```python
from build123d import *

# Parameters (mm, degrees)
BOSS_EXTRUDE1_DEPTH  = 12.5
CUT_EXTRUDE1_START   = -10
SKETCH2_W            = 31
SKETCH2_H            = 10
CUT_EXTRUDE1_DEPTH   = 161.165360752
CUT_EXTRUDE2_DEPTH   = 10
CUT_EXTRUDE3_DEPTH   = 2
FILLET3_R            = 2
FILLET3_OF_MIRROR2_R = 2
SKETCH6_R            = 3
CUT_EXTRUDE5_DEPTH   = 164.267418673
FILLET4_R            = 3
FILLET4_OF_MIRROR3_R = 3


with BuildPart() as part:
    # Sketch1 → Boss-Extrude1 (new, symmetric)
    with BuildSketch(Plane(origin=(0, 0, 0), x_dir=(1, 0, 0), z_dir=(0, 1, 0))):
        Polygon((0, 120), (10, 120), (120, 10), (120, 0), (85, 0), (85, 9.644660941), (9.644660941, 85), (0, 85), align=None)
    extrude(amount=BOSS_EXTRUDE1_DEPTH, both=True)

    # Sketch2 → Cut-Extrude1 (cut, through all)
    with BuildSketch(Plane.XY.offset(CUT_EXTRUDE1_START)):
        with Locations((104.5, 0)):
            Rectangle(SKETCH2_W, SKETCH2_H)
    cut_extrude1 = extrude(amount=-CUT_EXTRUDE1_DEPTH, mode=Mode.SUBTRACT)

    # Sketch3 → Cut-Extrude2 (cut)
    with BuildSketch(Plane.XZ.offset(12.5)):
        Polygon((57.505379907, -44.210348845), (85, -16.715728753), (85, -37.928932188), align=None)
        Polygon((16.715728753, -85), (37.928932188, -85), (44.210348845, -57.505379907), align=None)
        Polygon((44.576447719, -78.352484469), (78.352484469, -44.576447719), (50.857864376, -50.857864376), align=None)
    cut_extrude2 = extrude(amount=-CUT_EXTRUDE2_DEPTH, mode=Mode.SUBTRACT)

    # Sketch4 → Cut-Extrude3 (cut)
    with BuildSketch(Plane.XZ.offset(12.5)):
        Polygon((5, -90), (32.928932188, -90), (7.928932188, -115), (5, -115), align=None)
        Polygon((115, -5), (90, -5), (90, -32.928932188), (115, -7.928932188), align=None)
    cut_extrude3 = extrude(amount=-CUT_EXTRUDE3_DEPTH, mode=Mode.SUBTRACT)

    # Fillet3
    fillet3_edges = [part.edges().sort_by_distance(p)[0] for p in [
        (16.715728753, -7.5, -85),
        (44.210348845, -7.5, -57.505379907),
        (37.928932188, -7.5, -85),
        (50.857864376, -7.5, -50.857864376),
        (78.352484469, -7.5, -44.576447719),
        (44.576447719, -7.5, -78.352484469),
        (85, -7.5, -37.928932188),
        (57.505379907, -7.5, -44.210348845),
        (85, -7.5, -16.715728753),
        (5, -11.5, -115),
        (5, -11.5, -90),
        (32.928932188, -11.5, -90),
        (7.928932188, -11.5, -115),
        (90, -11.5, -32.928932188),
        (90, -11.5, -5),
        (115, -11.5, -5),
        (115, -11.5, -7.928932188),
    ]]
    fillet(fillet3_edges, radius=FILLET3_R)

    # Mirror2: Cut-Extrude2, Cut-Extrude3 across plane
    add(cut_extrude2.mirror(Plane.ZX), mode=Mode.SUBTRACT)
    add(cut_extrude3.mirror(Plane.ZX), mode=Mode.SUBTRACT)

    # Fillet3 of Mirror2
    fillet3_of_mirror2_edges = [part.edges().sort_by_distance(p)[0] for p in [
        (16.715728753, 7.5, -85),
        (44.210348845, 7.5, -57.505379907),
        (37.928932188, 7.5, -85),
        (50.857864376, 7.5, -50.857864376),
        (78.352484469, 7.5, -44.576447719),
        (44.576447719, 7.5, -78.352484469),
        (85, 7.5, -37.928932188),
        (57.505379907, 7.5, -44.210348845),
        (85, 7.5, -16.715728753),
        (5, 11.5, -115),
        (5, 11.5, -90),
        (32.928932188, 11.5, -90),
        (7.928932188, 11.5, -115),
        (90, 11.5, -32.928932188),
        (90, 11.5, -5),
        (115, 11.5, -5),
        (115, 11.5, -7.928932188),
    ]]
    fillet(fillet3_of_mirror2_edges, radius=FILLET3_OF_MIRROR2_R)

    # Sketch6 → Cut-Extrude5 (cut, through all)
    with BuildSketch(Plane(origin=(0, 0, -10), x_dir=(-1, 0, 0), z_dir=(0, 0, -1))):
        with Locations((-113.5, 0)):
            Circle(SKETCH6_R)
        with Locations((-95.5, 0)):
            Circle(SKETCH6_R)
    cut_extrude5 = extrude(amount=-CUT_EXTRUDE5_DEPTH, mode=Mode.SUBTRACT)

    # Fillet4
    fillet4_edges = [part.edges().sort_by_distance(p)[0] for p in [
        (89, -5, -25.5),
        (89, 5, -25.5),
    ]]
    fillet(fillet4_edges, radius=FILLET4_R)

    # Mirror3: Cut-Extrude1, Cut-Extrude5 across plane
    add(cut_extrude1.mirror(Plane(origin=(0, 0, 0), x_dir=(-0.7071067811865475, 0, 0.7071067811865477), z_dir=(0.7071067811865476, 0, 0.7071067811865475))), mode=Mode.SUBTRACT)
    add(cut_extrude5.mirror(Plane(origin=(0, 0, 0), x_dir=(-0.7071067811865475, 0, 0.7071067811865477), z_dir=(0.7071067811865476, 0, 0.7071067811865475))), mode=Mode.SUBTRACT)

    # Fillet4 of Mirror3
    fillet4_of_mirror3_edges = [part.edges().sort_by_distance(p)[0] for p in [
        (25.5, -5, -89),
        (25.5, 5, -89),
    ]]
    fillet(fillet4_of_mirror3_edges, radius=FILLET4_OF_MIRROR3_R)


solid = part.part
```
CAD build for the part. Positions are in the model's coordinates, mm. A direction names the side the tool comes from. Round coordinates to 2 decimals unless told otherwise and drop trailing zeros. Order: outer loops, then holes, each group sorted by start corner. A loop starts at its lowest first (then second) coordinate and runs counter-clockwise, first axis right, second up.
Item 1: Saw through at A-A on y = 6.75. Write the cut outline in (x, z), then the cut area to 3 significant figures.
Item 2: Saw through at C-C on x = 95.5. Write the cut outline in (y, z).
Item 3: Saw through at B-B on z = -95.5. Write the cut outline in (x, y).
Item 4: Tool access for faces 5 (the face through (120, 0, -5)), 6 (the face through (5, 0, -85)), 7 (the face through (73.795, 7.43, -47.137)), 8 (the face through (103.77, -11.51, -19.16)), 9 (the face through (5.07, 0.9, -110.64)): list every direction of +Z, -Z, +X, -X, +Y, -Y with a clear straight run to the whole face (end or side of a thin tool).
Item 5: Pin check, flat tips, straight feed: pin 1 (8.5 mm diameter, centred on x = 17, z = -103, fed in from +Y); pin 2 (4 mm diameter, centred on x = 88, y = 3, fed in from -Z); pin 3 (1 mm diameter, centred on y = -11.5, z = -19.5, fed in from +X); pin 4 (1.6 mm diameter, centred on x = 106.5, y = 11, fed in from -Z). Stop position of each tip, or through.
Item 6: Probe line 1 along Z through (x, y) = (7.5, 0); line 2 along Y through (x, z) = (95.5, -4.5); line 3 along Y through (x, z) = (113, -11). List the from-to ranges inside material, lowest first.
Item 7: Mould opens along Z. For faces 1 (the face through (83.8, -7.43, -19.71)), 2 (the face through (64, 0, -66)), 3 (the face through (0, 0, -102)), 4 (the face through (73.795, -7.43, -47.137)) say: pulls with the +Z half, pulls with the -Z half, needs draft (parallel to the pull), parting line crosses it, or undercut.
Item 8: Saw through at D-D on z = -13. Write the cut outline in (x, y).
Reported:
1. outline: (0, -120) - (10, -120) - (120, -10) - (120, 0) - (85, 0) - (85, -9.64) - (9.64, -85) - (0, -85) - close; hole (20.13, -81.59) arc R2 ccw to (21.54, -85) - (36.33, -85) arc R2 ccw to (38.28, -83.45) - (42.66, -64.28) arc R2 ccw to (39.3, -62.42) - close; hole (46.12, -71.58) arc R2 ccw to (49.49, -73.44) - (73.44, -49.49) arc R2 ccw to (71.58, -46.12) - (52.08, -50.58) arc R2 ccw to (50.58, -52.08) - close; hole (62.42, -39.3) arc R2 ccw to (64.28, -42.66) - (83.45, -38.28) arc R2 ccw to (85, -36.33) - (85, -21.54) arc R2 ccw to (81.59, -20.13) - close
1. area: 3,070 mm2
2. outline: (-12.5, -34.5) - (-5, -34.5) - (-5, -10) - (-3, -10) - (-3, 0) - (-12.5, 0) - (-12.5, -5) - (-10.5, -5) - (-10.5, -27.43) - (-12.5, -27.43) - close; (3, -10) - (5, -10) - (5, -34.5) - (12.5, -34.5) - (12.5, -27.43) - (10.5, -27.43) - (10.5, -5) - (12.5, -5) - (12.5, 0) - (3, 0) - close
3. outline: (0, -12.5) - (5, -12.5) - (5, -10.5) - (27.43, -10.5) - (27.43, -12.5) - (34.5, -12.5) - (34.5, -5) - (10, -5) - (10, -3) - (0, -3) - close; (0, 3) - (10, 3) - (10, 5) - (34.5, 5) - (34.5, 12.5) - (27.43, 12.5) - (27.43, 10.5) - (5, 10.5) - (5, 12.5) - (0, 12.5) - close
4. face 5: +Z, -Z, +X, +Y, -Y
4. face 6: +Z, -X, +Y, -Y
4. face 7: +Y
4. face 8: -Y
4. face 9: +X, -X
5. pin 1: stops at y = 12.5
5. pin 2: stops at z = -44
5. pin 3: stops at x = 111
5. pin 4: stops at z = -24.3
6. line 1: z = -120 to -116.5, -110.5 to -98.5, -92.5 to -85
6. line 2: y = -12.5 to -3, 3 to 12.5
6. line 3: y = -12.5 to -5, 5 to 12.5
7. face 1: undercut
7. face 2: pulls with the -Z half
7. face 3: needs draft
7. face 4: undercut
8. outline: (81.64, -12.5) - (90, -12.5) - (90, -10.5) - (109.93, -10.5) - (109.93, -12.5) - (117, -12.5) - (117, -5) - (92, -5) arc R3 cw to (89, -2) - (89, 2) arc R3 cw to (92, 5) - (117, 5) - (117, 12.5) - (109.93, 12.5) - (109.93, 10.5) - (90, 10.5) - (90, 12.5) - (81.64, 12.5) - close
